from build123d import *

# Parameters (mm, degrees)
SKETCH1_R               = 48.5
SKETCH1_R_2             = 1.5
SKETCH1_W               = 5
SKETCH1_H               = 15
BOSS_EXTRUDE1_DEPTH     = 4
SKETCH1_4_W             = 5
SKETCH1_4_H             = 15
BOSS_EXTRUDE2_DEPTH     = 15
FILLET1_R               = 2
EXTRUDE_THIN1_DEPTH     = 11
BOSS_EXTRUDE3_START     = 11
SKETCH3_4_R             = 10.1
BOSS_EXTRUDE3_DEPTH     = 11
CUT_EXTRUDE2_DEPTH      = 11
SKETCH8_R               = 1.5
CUT_EXTRUDE3_DEPTH      = 9
CUT_EXTRUDE4_DEPTH      = 110.483799158
CUT_EXTRUDE4_DEPTH_BACK = 110.483799158
SKETCH9_W               = 8
SKETCH9_H               = 4
SKETCH10_W              = 15
SKETCH10_H              = 10
CUT_EXTRUDE5_DEPTH      = 93.739106768
FILLET2_R               = 7.5
BOSS_EXTRUDE4_START     = 2.5
SKETCH11_R              = 1.5
BOSS_EXTRUDE4_DEPTH     = 2.5


with BuildPart() as part:
    # Sketch1 → Boss-Extrude1 (new body)
    with BuildSketch(Plane(origin=(0, 0, 0), x_dir=(1, 0, 0), z_dir=(0, 1, 0))):
        with Locations(Location((0, 0, 0), (0, 0, 270))):
            Circle(SKETCH1_R)
        with Locations(Location((7.5, 1.5, 0), (0, 0, 270))):
            Circle(SKETCH1_R_2, mode=Mode.SUBTRACT)
        with Locations(Location((-7.5, 1.5, 0), (0, 0, 270))):
            Circle(SKETCH1_R_2, mode=Mode.SUBTRACT)
        with Locations((-21, -6)):
            Rectangle(SKETCH1_W, SKETCH1_H, mode=Mode.SUBTRACT)
    extrude(amount=BOSS_EXTRUDE1_DEPTH)

    # Sketch1<4> → Boss-Extrude2 (add)
    with BuildSketch(Plane(origin=(0, 0, 0), x_dir=(1, 0, 0), z_dir=(0, 1, 0))):
        with Locations((-21, -6)):
            Rectangle(SKETCH1_4_W, SKETCH1_4_H)
    extrude(amount=BOSS_EXTRUDE2_DEPTH)

    # Fillet1
    fillet1_edges = [part.edges().sort_by_distance(p)[0] for p in [
        (-21, 15, -1.5),
        (-21, 15, 13.5),
    ]]
    fillet(fillet1_edges, radius=FILLET1_R)

    # Sketch3 → Extrude-Thin1 (add, symmetric)
    with BuildSketch(Plane.XY.offset(-16)):
        with BuildLine():
            Line((-33.5, 0), (-33.5, 14.02081119))
            ThreePointArc((-33.5, 14.02081119), (-32.433806578, 19.575001882), (-29.386795435, 24.339613696))
            Line((-29.386795435, 24.339613696), (1.569612084, 57))
            ThreePointArc((1.569612084, 57), (45.23729846, 52.625424101), (30.061304851, 11.446631432))
            ThreePointArc((30.061304851, 11.446631432), (28.251643763, 10.794728993), (26.5, 10))
            Line((26.5, 10), (26.5, 0))
            Line((26.5, 0), (16.5, 0))
            Line((16.5, 0), (16.5, 15.467006733))
            ThreePointArc((16.5, 15.467006733), (21.532603297, 18.690532933), (27.051891801, 20.983058074))
            ThreePointArc((27.051891801, 20.983058074), (36.759058885, 47.322646177), (8.827475707, 50.120798329))
            Line((8.827475707, 50.120798329), (-22.128931812, 17.460412025))
            ThreePointArc((-22.128931812, 17.460412025), (-23.144602193, 15.872208087), (-23.5, 14.02081119))
            Line((-23.5, 14.02081119), (-23.5, 0))
            Line((-23.5, 0), (-33.5, 0))
        make_face()
    extrude(amount=EXTRUDE_THIN1_DEPTH, both=True)

    # Sketch3<4> → Boss-Extrude3 (add)
    with BuildSketch(Plane.XY.offset(-16).offset(BOSS_EXTRUDE3_START)):
        with BuildLine():
            Line((-33.5, 0), (-33.5, 14.02081119))
            ThreePointArc((-33.5, 14.02081119), (-32.433806578, 19.575001882), (-29.386795435, 24.339613696))
            Line((-29.386795435, 24.339613696), (1.569612084, 57))
            ThreePointArc((1.569612084, 57), (45.23729846, 52.625424101), (30.061304851, 11.446631432))
            ThreePointArc((30.061304851, 11.446631432), (28.251643763, 10.794728993), (26.5, 10))
            Line((26.5, 10), (26.5, 0))
            Line((26.5, 0), (-33.5, 0))
        make_face()
        with Locations(Location((21.710183638, 37.910215363, 0), (0, 0, 180))):
            Circle(SKETCH3_4_R, mode=Mode.SUBTRACT)
    extrude(amount=-BOSS_EXTRUDE3_DEPTH)

    # Sketch5 → Cut-Extrude2 (cut)
    with BuildSketch(Plane(origin=(0, 0, -27), x_dir=(-1, 0, 0), z_dir=(0, 0, -1))):
        with BuildLine():
            Line((-16.5, 4), (25.5, 4))
            ThreePointArc((25.5, 4), (24.270182893, 20.088149503), (16.096969308, 34))
            Line((16.096969308, 34), (-3.746971171, 54.936239499))
            ThreePointArc((-3.746971171, 54.936239499), (-42.693826587, 51.034590724), (-29.158480936, 14.307559424))
            ThreePointArc((-29.158480936, 14.307559424), (-21.844187603, 10.363500889), (-16.5, 4))
        make_face()
    extrude(amount=-CUT_EXTRUDE2_DEPTH, mode=Mode.SUBTRACT)

    # Sketch8 → Cut-Extrude3 (cut)
    with BuildSketch(Plane(origin=(0, 0, -16), x_dir=(-1, 0, 0), z_dir=(0, 0, -1))):
        with Locations((-35.648743891, 43.079019683)):
            Circle(SKETCH8_R)
        with Locations((-29.220867794, 50.739464115)):
            Circle(SKETCH8_R)
        with Locations(Location((7.549265476, 19.88565885, 0), (0, 0, 180))):
            Circle(SKETCH8_R)
        with Locations(Location((1.121389379, 12.225214418, 0), (0, 0, 180))):
            Circle(SKETCH8_R)
        Polygon((-37.207336219, 36.554390196), (-23.066008806, 53.407367944), (9.107857805, 26.410288337), (-5.033469608, 9.557310589), align=None)
    extrude(amount=-CUT_EXTRUDE3_DEPTH, mode=Mode.SUBTRACT)

    # Sketch9 → Cut-Extrude4 (cut, two sides: drawn at the far end of the back side and taken through both)
    with BuildSketch(Plane.ZY.offset(23.5).offset(-CUT_EXTRUDE4_DEPTH_BACK)):
        with Locations((6, 9)):
            Rectangle(SKETCH9_W, SKETCH9_H)
    extrude(amount=CUT_EXTRUDE4_DEPTH + CUT_EXTRUDE4_DEPTH_BACK, mode=Mode.SUBTRACT)

    # Sketch10 → Cut-Extrude5 (cut, through all)
    with BuildSketch(Plane(origin=(0, 4, 0), x_dir=(1, 0, 0), z_dir=(0, 1, 0))):
        with Locations((-10.5, 29)):
            Rectangle(SKETCH10_W, SKETCH10_H)
    extrude(amount=-CUT_EXTRUDE5_DEPTH, mode=Mode.SUBTRACT)

    # Fillet2
    fillet2_edges = [part.edges().sort_by_distance(p)[0] for p in [
        (26.5, 10, -16),
    ]]
    fillet(fillet2_edges, radius=FILLET2_R)

    # Sketch11 → Boss-Extrude4 (add)
    with BuildSketch(Plane(origin=(0, 0, -16), x_dir=(-1, 0, 0), z_dir=(0, 0, -1)).offset(BOSS_EXTRUDE4_START)):
        with BuildLine():
            Line((-16.5, 4), (25.5, 4))
            ThreePointArc((25.5, 4), (24.270182893, 20.088149503), (16.096969308, 34))
            Line((16.096969308, 34), (-3.746971171, 54.936239499))
            ThreePointArc((-3.746971171, 54.936239499), (-42.693826587, 51.034590724), (-29.158480936, 14.307559424))
            ThreePointArc((-29.158480936, 14.307559424), (-21.844187603, 10.363500889), (-16.5, 4))
        make_face()
        with Locations((1.121389379, 12.225214418)):
            Circle(SKETCH11_R, mode=Mode.SUBTRACT)
        with Locations((7.549265476, 19.88565885)):
            Circle(SKETCH11_R, mode=Mode.SUBTRACT)
        with Locations((-35.648743891, 43.079019683)):
            Circle(SKETCH11_R, mode=Mode.SUBTRACT)
        with Locations((-29.220867794, 50.739464115)):
            Circle(SKETCH11_R, mode=Mode.SUBTRACT)
        Polygon((-5.033469608, 9.557310589), (9.107857805, 26.410288337), (-23.066008806, 53.407367944), (-37.207336219, 36.554390196), align=None, mode=Mode.SUBTRACT)
    extrude(amount=-BOSS_EXTRUDE4_DEPTH)


solid = part.part
Geometry: final body of the model. Coordinates: model frame, mm. A direction names the side the tool comes from. Give positions to 0.01 mm unless a question says otherwise; leave off trailing zeros. Loops run counter-clockwise (first coordinate to the right, second up) from the corner with the lowest first, then second, coordinate; pieces in that order, holes last. Notation, with made-up numbers: (20.25, 2.25) -> (77.25, 2.25) arc R13 cw to (77.25, 17.25) -> close; hole circle Ø8 at (57.5, 21). An arc over 180 degrees is marked (long way). Put each result on its own line as item: value.
1. Cut plane B-B (y = 46). Return the cut outline in (x, z).
Taken from the geometry:
outline: (-8.86, -27) -> (-4.72, -27) -> (-4.72, -18.5) -> (14.24, -18.5) -> (14.24, -7) -> (15.66, -7) -> (15.66, -5) -> (-8.86, -5) -> close; (27.76, -7) -> (29.28, -7) -> (29.28, -18.5) -> (45.1, -18.5) -> (45.1, -27) -> (48.25, -27) -> (48.25, -5) -> (27.76, -5) -> close
2. Set-up query: faces 4 (the flat face through (-21, 11, 6)), 5 (the flat face through (1, 4, -1)), 6 (the flat face through (-21, 8, -1.5)), 7 (the cylindrical face through (29.416, 52.227, -12.83)). Return all of +Z, -Z, +X, -X, +Y, -Y with unobstructed straight access to the full face (end or side cutting, diameter ignored); none if empty.
Taken from the geometry:
face 4: +X, -X
face 5: none
face 6: +X, -X, +Y
face 7: -Z
3. Cut plane A-A (x = 7.5). Return the cut outline in (y, z).
Taken from the geometry:
outline: (0, -47.92) -> (4, -47.92) -> (4, -18.5) -> (11.63, -18.5) -> (11.63, -7) -> (40.35, -7) -> (40.35, -18.5) -> (58.17, -18.5) -> (58.17, -27) -> (61.75, -27) -> (61.75, -5) -> (4, -5) -> (4, -3) -> (0, -3) -> close; (0, 0) -> (4, 0) -> (4, 47.92) -> (0, 47.92) -> close
4. Ray query, line 1 along X through (y, z) = (3.2, -1.5); line 2 along X through (y, z) = (1, -1); line 3 along Z through (x, y) = (-22.5, 6). Return the intervals inside material, ascending. Write a range as [from, to].
Taken from the geometry:
line 1: x = [-48.48, -9], [-6, 6], [9, 48.48]
line 2: x = [-48.49, -8.91], [-6.09, 6.09], [8.91, 48.49]
line 3: z = [-18.5, -5], [-1.5, 13.5]
5. Cut plane C-C (x = -7.5). Return the cut outline in (y, z).
Taken from the geometry:
outline: (0, -47.92) -> (4, -47.92) -> (4, -34) -> (0, -34) -> close; (0, -24) -> (4, -24) -> (4, -18.5) -> (18.39, -18.5) -> (18.39, -7) -> (21.38, -7) -> (21.38, -18.5) -> (24.49, -18.5) -> (24.49, -7) -> (27.76, -7) -> (27.76, -18.5) -> (43.07, -18.5) -> (43.07, -27) -> (47.43, -27) -> (47.43, -5) -> (4, -5) -> (4, -3) -> (0, -3) -> close; (0, 0) -> (4, 0) -> (4, 47.92) -> (0, 47.92) -> close
6. Pin query (flat end, axial travel): P1, Ø3, axis at x = -13, z = -13.5, coming from the +Y side; P2, Ø3, axis at x = -2, y = 52.5, coming from the -Z side; P3, Ø3.5, axis at y = 7, z = 6.5, coming from the -X side. Return the tip coordinate at first contact, or that it passes through.
Taken from the geometry:
P1: stops at y = 43.21
P2: stops at z = -27
P3: stops at x = -23.5
7. Pull-direction query (Y, two-part tool) for faces 1 (the cylindrical face through (42.35, 51.57, -22.81)), 2 (the flat face through (-14.125, 40.441, -15.846)), 3 (the cylindrical face through (6.036, 1.972, -1.825)); classes: released by +Y, released by -Y, zero draft, split by the parting line, or undercut.
Taken from the geometry:
face 1: undercut
face 2: released by +Y
face 3: zero draft
8. Cut plane D-D (x = -20). Return the cut outline in (y, z), plus the area to 3 significant figures.
Taken from the geometry:
outline: (0, -44.18) -> (4, -44.18) -> (4, -18.5) -> (29.08, -18.5) -> (29.08, -27) -> (34.24, -27) -> (34.24, -5) -> (4, -5) -> (4, -1.5) -> (13, -1.5) arc R2 ccw to (15, 0.5) -> (15, 11.5) arc R2 ccw to (13, 13.5) -> (4, 13.5) -> (4, 44.18) -> (0, 44.18) -> close; hole (7, 2) -> (11, 2) -> (11, 10) -> (7, 10) -> close
area: 937 mm2
